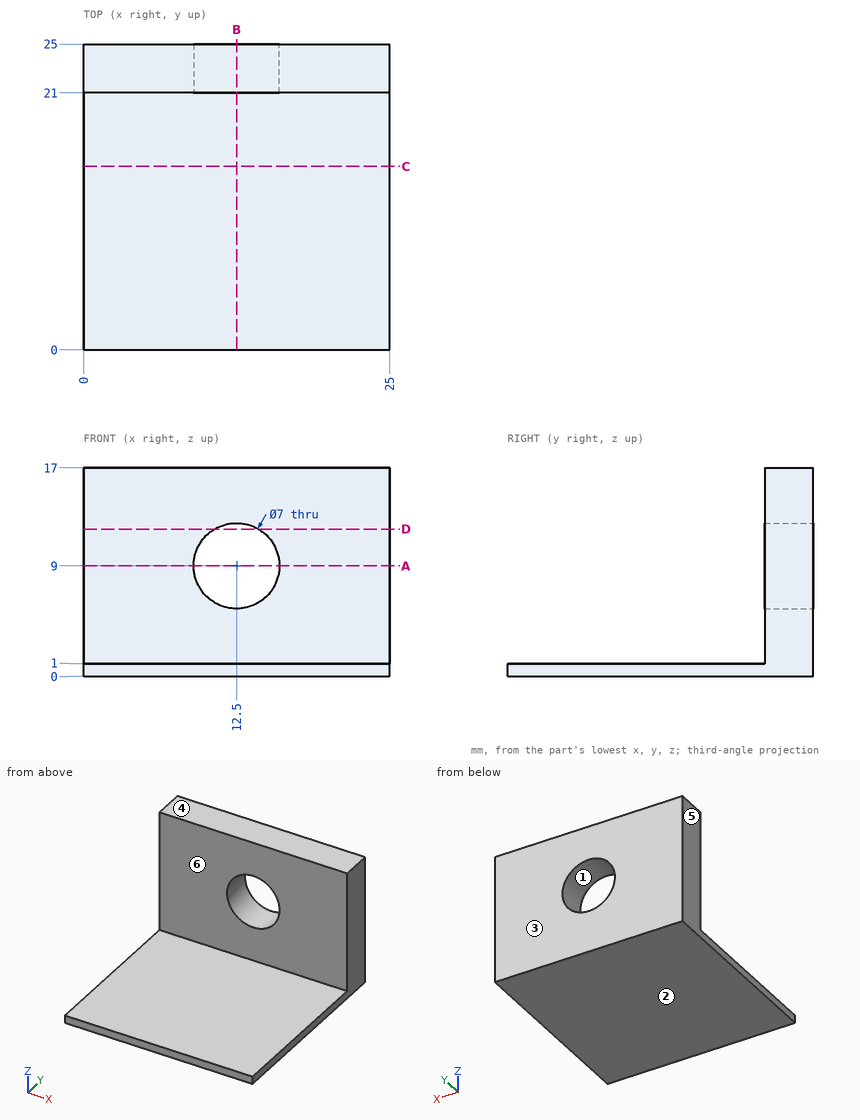
Answer from the drawing. Dimensions are ordinates in mm from the lowest x, y and z of the part. A direction names the side the tool comes from. Coordinates: 2 decimals unless noted, no trailing zeros. Loops run counter-clockwise (first coordinate to the right, second up) from the corner with the lowest first, then second, coordinate; pieces in that order, holes last. Notation, with made-up numbers: (38.5, 41.5) -> (53.5, 41.5) arc R31 cw to (53.5, 76.5) -> close; hole circle Ø1 at (-26, 20.5). An arc over 180 degrees is marked (long way). Return JSON: item names as keys, results as strings.
Item 1: Find section D-D (z = 12). Determine the outline of the cut face in (x, y).
Answers:
{"outline": "(0, 21) -> (10.7, 21) -> (10.7, 25) -> (0, 25) -> close; (14.3, 21) -> (25, 21) -> (25, 25) -> (14.3, 25) -> close"}
Item 2: Find section B-B (x = 12.5). Determine the outline of the cut face in (y, z).
Answers:
{"outline": "(0, 0) -> (25, 0) -> (25, 5.5) -> (21, 5.5) -> (21, 1) -> (0, 1) -> close; (21, 12.5) -> (25, 12.5) -> (25, 17) -> (21, 17) -> close"}
Item 3: Find section C-C (y = 15). Determine the outline of the cut face in (x, z), plus the area to 3 significant figures.
Answers:
{"outline": "(0, 0) -> (25, 0) -> (25, 1) -> (0, 1) -> close", "area": "25.0 mm2"}
Item 4: Find the intervals of material crossed by probe 1 along Z at (x, y) = (12.5, 24.1); probe 2 along Z at (x, y) = (16.75, 10); probe 3 along Y at (x, z) = (20, 11.25), in increasing order.
Answers:
{"probe 1": "z = 0 to 5.5, 12.5 to 17", "probe 2": "z = 0 to 1", "probe 3": "y = 21 to 25"}
Item 5: Find section A-A (z = 9). Determine the outline of the cut face in (x, y).
Answers:
{"outline": "(0, 21) -> (9, 21) -> (9, 25) -> (0, 25) -> close; (16, 21) -> (25, 21) -> (25, 25) -> (16, 25) -> close"}
Item 6: For a pull along Z with two mould halves and no side action, classify the marked faces 1, 2, 3 and 4 as +Z half, -Z half, draft (parallel to the pull), parting line (faces both ways), or undercut.
Answers:
{"face 1": "undercut", "face 2": "-Z half", "face 3": "draft", "face 4": "+Z half"}
Item 7: Flat-ended cylindrical pins translate along their axes: P1, Ø9, axis at x = 12.5, z = 9, coming from the +Y side; P2, Ø3, axis at x = 12.5, y = 9, coming from the +Z side; P3, Ø1, axis at x = 19.5, z = 10, coming from the -Y side. Find the tip coordinate at first contact, or state that the pin passes through.
Answers:
{"P1": "stops at y = 25", "P2": "stops at z = 1", "P3": "stops at y = 21"}
Item 8: For the marked faces 5 and 6, determine the directions among +Z, -Z, +X, -X, +Y, -Y from which every point of the face is accessible in a straight line to the end or side of a thin tool.
Answers:
{"face 5": "+Z, -Z, -X, +Y, -Y", "face 6": "+Z, +X, -X, -Y"}
